from build123d import *

# Parameters (mm, degrees)
ESQUISSE1_W             = 40
ESQUISSE1_H             = 20
BOSS_EXTRU_1_DEPTH      = 10
ESQUISSE2_R             = 3.1
ENL_V_MAT_EXTRU_1_DEPTH = 10
ESQUISSE3_W             = 40
ESQUISSE3_H             = 2.1
ENL_V_MAT_EXTRU_2_DEPTH = 31
ESQUISSE4_R             = 2.05
ENL_V_MAT_EXTRU_3_DEPTH = 25.494897428


with BuildPart() as part:
    # Esquisse1 → Boss.-Extru.1 (new body)
    with BuildSketch(Plane.XY):
        Rectangle(ESQUISSE1_W, ESQUISSE1_H)
    extrude(amount=BOSS_EXTRU_1_DEPTH)

    # Esquisse2 → Enlèv. mat.-Extru.1 (cut)
    with BuildSketch(Plane.XY.offset(10)):
        Circle(ESQUISSE2_R)
    extrude(amount=-ENL_V_MAT_EXTRU_1_DEPTH, mode=Mode.SUBTRACT)

    # Esquisse3 → Enlèv. mat.-Extru.2 (cut, through all)
    with BuildSketch(Plane(origin=(0, -10, 0), x_dir=(-1, 0, 0), z_dir=(0, -1, 0))):
        with Locations((20, -5)):
            Rectangle(ESQUISSE3_W, ESQUISSE3_H)
    extrude(amount=-ENL_V_MAT_EXTRU_2_DEPTH, mode=Mode.SUBTRACT)

    # Esquisse4 → Enlèv. mat.-Extru.3 (cut, through all)
    with BuildSketch(Plane(origin=(0, 0, 0), x_dir=(-1, 0, 0), z_dir=(0, 0, -1))):
        with Locations((16, 6)):
            Circle(ESQUISSE4_R)
        with Locations((4, 6)):
            Circle(ESQUISSE4_R)
        with Locations((4, -6)):
            Circle(ESQUISSE4_R)
        with Locations((16, -6)):
            Circle(ESQUISSE4_R)
    extrude(amount=-ENL_V_MAT_EXTRU_3_DEPTH, mode=Mode.SUBTRACT)


solid = part.part
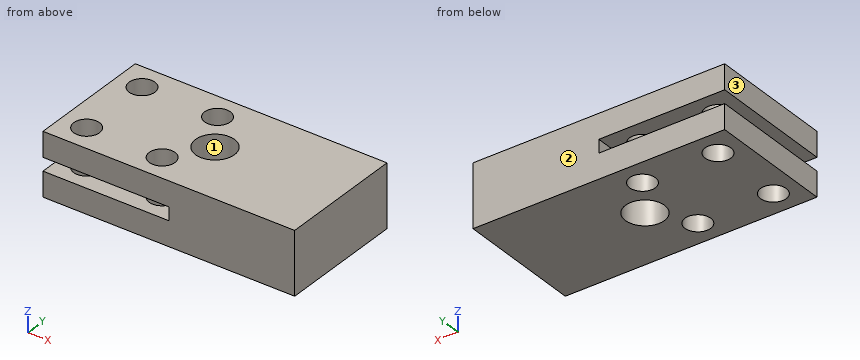
Source: CAD feature listing. Evaluate the final solid. Frame: model axes, mm. Face numbers are marked on the shaded views. Give positions to 0.01 mm unless a question says otherwise; leave off trailing zeros. Write each loop counter-clockwise with the first axis right and the second up, starting at its lowest first coordinate (ties: lowest second). Pieces come first, ordered by that corner, then holes. Notation, with made-up numbers: (88.5, -21) - (104.5, -21) arc R25 ccw to (104.5, 11) - close; hole circle Ø6 at (63, 62). An arc over 180 degrees is marked (long way). Write item = value, one per line. Start each with the question number.
Q1. Cut plane D-D, the plane x = -4. Return loops of the section in (y, z), then the cut area to 3 significant figures.
Q2. Cut plane B-B, the plane y = 0. Return loops of the section in (x, z).
Q3. Cut plane C-C, the plane z = 7.5. Return loops of the section in (x, y), then the cut area to 3 significant figures.
Q4. Cut plane A-A, the plane x = -12. Return loops of the section in (y, z).
Q5. Draft query along X for the marked faces 1, 2 and 3. Return one class per face: +X half, -X half, draft (parallel to the pull), parting line (faces both ways), or undercut.
Q6. Pin query (flat end, axial travel): pin 1 Ø1 at (y, z) = (-7.5, 4.5) entering from -X. Return the tip coordinate at first contact, or that it passes through.
Q7. Material intervals for probe 1 along Y at (x, z) = (-4, 8.95); probe 2 along Z at (x, y) = (-14, -1); probe 3 along Y at (x, z) = (0, 3.75), sorted ascending.
Computed values:
q1.outline = (-10, 0) - (-8.05, 0) - (-8.05, 3.95) - (-10, 3.95) - close; (-10, 6.05) - (-8.05, 6.05) - (-8.05, 10) - (-10, 10) - close; (-3.95, 0) - (3.95, 0) - (3.95, 3.95) - (-3.95, 3.95) - close; (-3.95, 6.05) - (3.95, 6.05) - (3.95, 10) - (-3.95, 10) - close; (8.05, 0) - (10, 0) - (10, 3.95) - (8.05, 3.95) - close; (8.05, 6.05) - (10, 6.05) - (10, 10) - (8.05, 10) - close
q1.area = 93.2 mm²
q2.outline = (-20, 0) - (-3.1, 0) - (-3.1, 3.95) - (-20, 3.95) - close; (-20, 6.05) - (-3.1, 6.05) - (-3.1, 10) - (-20, 10) - close; (3.1, 0) - (20, 0) - (20, 10) - (3.1, 10) - close
q3.outline = (-20, -10) - (20, -10) - (20, 10) - (-20, 10) - close; hole circle Ø4.1 at (-16, -6); hole circle Ø4.1 at (-16, 6); hole circle Ø4.1 at (-4, -6); hole circle Ø4.1 at (-4, 6); hole circle Ø6.2 at (0, 0)
q3.area = 717 mm²
q4.outline = (-10, 0) - (10, 0) - (10, 3.95) - (-10, 3.95) - close; (-10, 6.05) - (10, 6.05) - (10, 10) - (-10, 10) - close
q5.face_1 = undercut
q5.face_2 = draft
q5.face_3 = -X half
q6.pin_1 = 0
q7.probe_1 = -10 to -8.05, -3.95 to 3.95, 8.05 to 10
q7.probe_2 = 0 to 3.95, 6.05 to 10
q7.probe_3 = -10 to -3.1, 3.1 to 10
